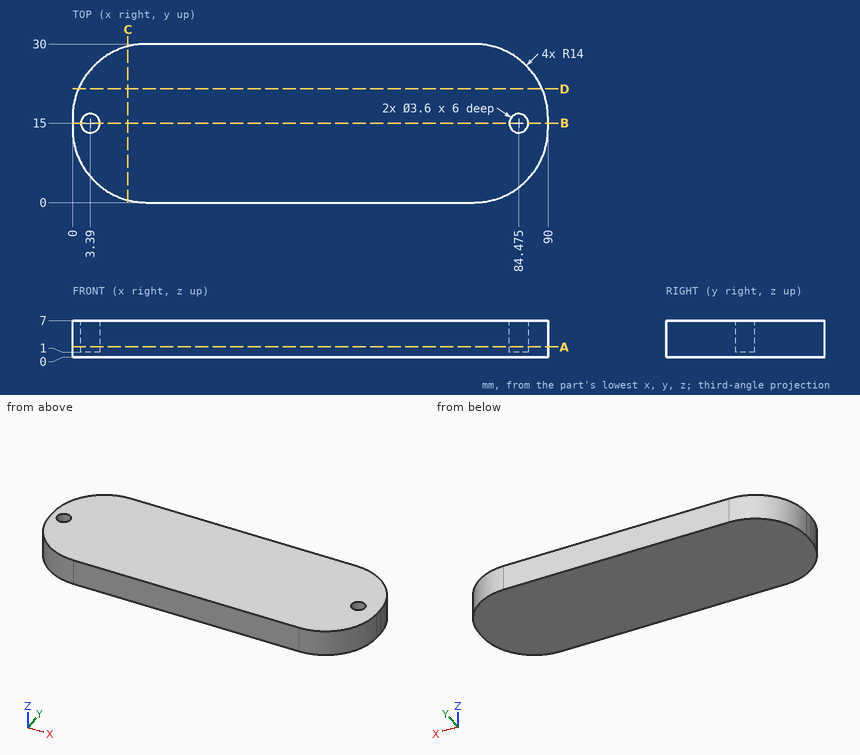
The drawing under review shows one solid part. Ordinate dimensions are in mm from its lowest x, y, z. Coordinates: 2 decimals unless noted, no trailing zeros. Write each loop counter-clockwise with the first axis right and the second up, starting at its lowest first coordinate (ties: lowest second). Pieces come first, ordered by that corner, then holes. Notation, with made-up numbers: (25.5, -35) -> (56.5, -35) arc R12 ccw to (56.5, -15) -> close; hole circle Ø2 at (14.25, 37.5). An arc over 180 degrees is marked (long way). Write each question's results on one line, items separated by ' | '. Start each with the question number.
1) Consider section A-A (z = 2). Write out the cut boundary in (x, y) (1 decimal).
2) Consider section B-B (y = 15). Write out the cut boundary in (x, z) (1 decimal), plus the area to 3 significant figures.
3) Wall thickness on L1, parallel to Y at x = 83.5, z = 2 (1 decimal); L2, parallel to X at y = 19, z = 3 (1 decimal); L3, parallel to Y at x = 8, z = 4.5: over which ranges is each line inside the solid? List them lowest first. Write a range as [from, to].
4) Consider section C-C (x = 10.5). Write out the cut boundary in (y, z) (1 decimal), plus the area to 3 significant figures.
5) Consider section D-D (y = 21.5). Write out the cut boundary in (x, z) (1 decimal), plus the area to 3 significant figures.
6) Insertion check: pin 1 (4 mm diameter, centred on x = 84.47, y = 15, fed in from +Z). The pin has a flat end and moves straight along its axis. Give the tip position at first contact, or say it passes through.
Geometry says:
1) outline: (0, 14) arc R14 ccw to (14, 0) -> (76, 0) arc R14 ccw to (90, 14) -> (90, 16) arc R14 ccw to (76, 30) -> (14, 30) arc R14 ccw to (0, 16) -> close; hole circle Ø3.6 at (3.4, 15); hole circle Ø3.6 at (84.5, 15)
2) outline: (0, 0) -> (90, 0) -> (90, 7) -> (86.3, 7) -> (86.3, 1) -> (82.7, 1) -> (82.7, 7) -> (5.2, 7) -> (5.2, 1) -> (1.6, 1) -> (1.6, 7) -> (0, 7) -> close | area: 587 mm^2
3) L1: [2.2, 13.5], [16.5, 27.8] | L2: [0.3, 89.7] | L3: [1.35, 28.65]
4) outline: (0.4, 0) -> (29.6, 0) -> (29.6, 7) -> (0.4, 7) -> close | area: 204 mm^2
5) outline: (1.1, 0) -> (88.9, 0) -> (88.9, 7) -> (1.1, 7) -> close | area: 614 mm^2
6) pin 1: z = 7
